Here's how the part is built. I have some questions about the finished solid (model axes, mm). Round coordinates to 2 decimals unless told otherwise and drop trailing zeros. Write each loop counter-clockwise with the first axis right and the second up, starting at its lowest first coordinate (ties: lowest second). Pieces come first, ordered by that corner, then holes. Notation, with made-up numbers: M -26,-28 L 11,-28 A24 ccw 11,11 Z; hole C 22.25,42.25 d10. An arc over 180 degrees is marked long. Use one line per item in the form item = value. Start each with the question number.
Q1. I'm going to push a flat-ended pin straight in: pin 1 Ø1 at (x, z) = (15.5, 2.5) entering from -Y. Where does the tip first touch, or does it pass through?
Q2. I want a section at B-B on y = 48. List the corners of the cut face in (x, z) for me (3 decimals), and give its area (3 significant figures).
Q3. I need wall thicknesses on line 1 along X through (y, z) = (-2.5, 0.8); line 2 along X through (y, z) = (40, 2.3); line 3 along Y through (x, z) = (-9, 1.8). Which ranges of each line are inside material? Lowest first, please. Write a range as from..to.
Q4. I want a section at C-C on z = 2.6. List the corners of the cut face in (x, y) for me.
Q5. I want a section at A-A on x = -16. List the corners of the cut face in (y, z) for me (3 decimals), and give its area (3 significant figures).
```python
from build123d import *

# Parameters (mm, degrees)
SKETCH1_R           = 69.85
SKETCH1_R_2         = 55.88
BOSS_EXTRUDE1_DEPTH = 3.175
SKETCH4_R           = 1.27
SKETCH4_R_2         = 2.54
CUT_EXTRUDE2_DEPTH  = 108.317012813


with BuildPart() as part:
    # Sketch1 → Boss-Extrude1 (new body)
    with BuildSketch(Plane.XY):
        with Locations((-8.548720341, -3.365444156)):
            Circle(SKETCH1_R)
        with Locations((-8.548720341, -3.365444156)):
            Circle(SKETCH1_R_2, mode=Mode.SUBTRACT)
    extrude(amount=BOSS_EXTRUDE1_DEPTH)

    # Sketch4 → Cut-Extrude2 (cut, through all)
    with BuildSketch(Plane(origin=(0, 0, 0), x_dir=(-1, 0, 0), z_dir=(0, 0, -1))):
        with Locations((8.548720341, 55.689555844)):
            Circle(SKETCH4_R)
        with Locations((8.548720341, -62.420444156)):
            Circle(SKETCH4_R)
        with Locations((-50.506279659, -3.365444156)):
            Circle(SKETCH4_R)
        with Locations((67.603720341, -3.365444156)):
            Circle(SKETCH4_R)
        with Locations((-33.658483428, 38.841759613)):
            Circle(SKETCH4_R_2)
        with Locations((50.75592411, -45.572647925)):
            Circle(SKETCH4_R_2)
    extrude(amount=-CUT_EXTRUDE2_DEPTH, mode=Mode.SUBTRACT)


solid = part.part
```
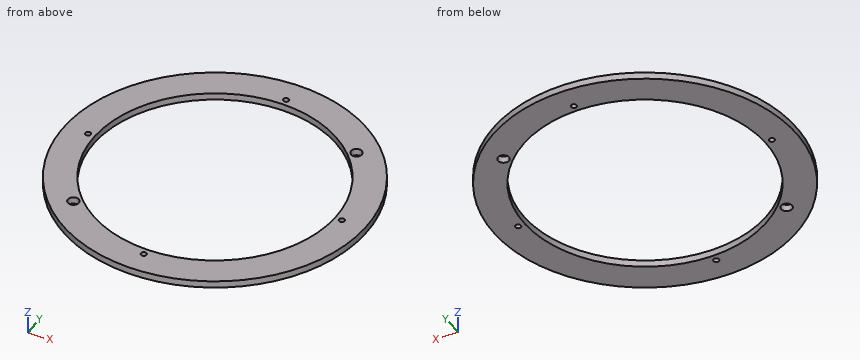
Reported:
q1.pin_1 = -69.13
q2.outline = M -55.884,0 L -30.552,0 L -30.552,3.175 L -55.884,3.175 Z; M 13.455,0 L 38.786,0 L 38.786,3.175 L 13.455,3.175 Z
q2.area = 161 mm^2
q3.line_1 = -78.39..-68.53, -66.67..-64.42, 47.32..49.58, 51.44..61.3
q3.line_2 = -63.31..-43.79, 26.69..31.4, 35.92..46.21
q3.line_3 = -73.21..-63.61, -61.23..-59.24, 52.51..54.5, 56.88..66.48
q4.outline = C -8.55,-3.37 d139.7; hole C -67.6,-3.37 d2.54; hole C -8.55,-3.37 d111.76; hole C -50.76,-45.57 d5.08; hole C -8.55,-62.42 d2.54; hole C -8.55,55.69 d2.54; hole C 33.66,38.84 d5.08; hole C 50.51,-3.37 d2.54
q5.outline = M -72.817,0 L -58.746,0 L -58.746,3.175 L -72.817,3.175 Z; M 52.016,0 L 66.086,0 L 66.086,3.175 L 52.016,3.175 Z
q5.area = 89.3 mm^2
